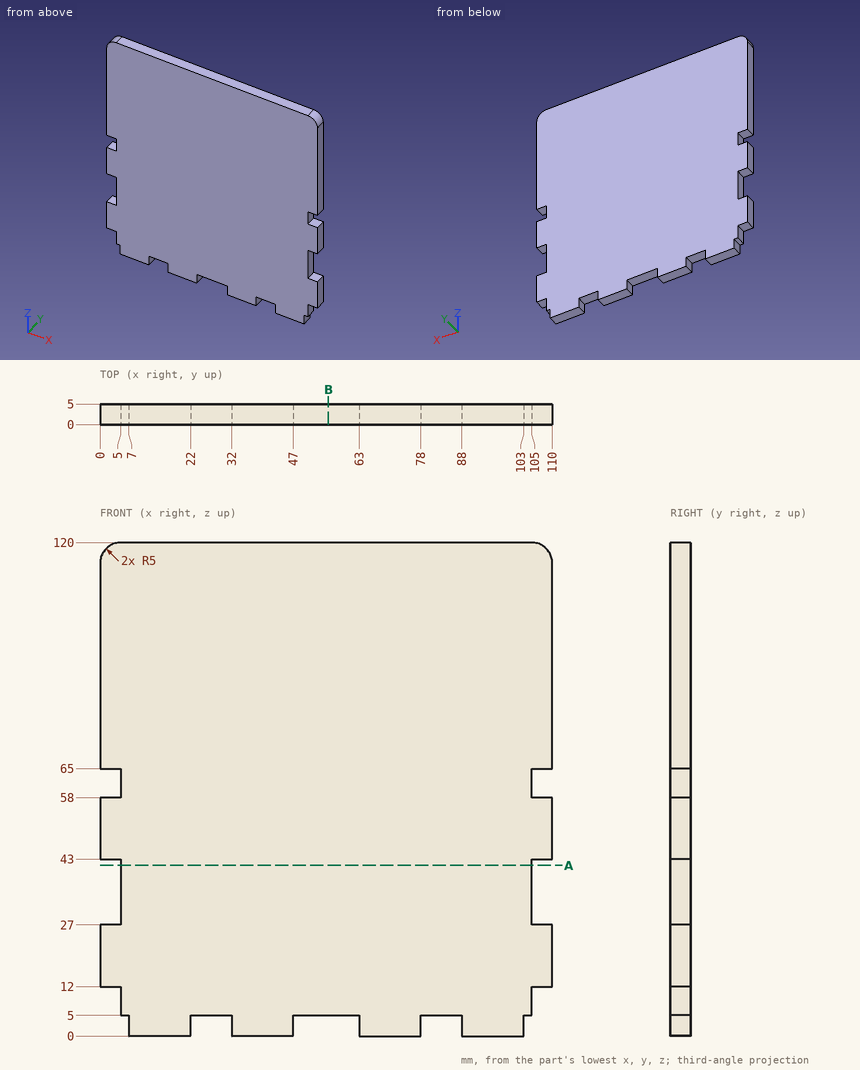
The figure shows three views and two pictorial views of one solid part (mm, origin at its lowest corner). Answer the questions. Give positions to 0.01 mm unless a question says otherwise; leave off trailing zeros. Loops run counter-clockwise (first coordinate to the right, second up) from the corner with the lowest first, then second, coordinate; pieces in that order, holes last. Notation, with made-up numbers: (41, 76) -> (68, 76) arc R18 cw to (68, 89) -> close; hole circle Ø2 at (51.25, -5.75). An arc over 180 degrees is marked (long way). Use a Markdown table: item, result. Add a question column.
1. Section A-A on z = 41.5 is taken. Determine the outline of the cut face in (x, y), and give its area (3 significant figures).
2. Flat-ended cylindrical pins translate along their axes: pin 1 Ø2.5 at (y, z) = (2.5, 3) entering from -X; pin 2 Ø1 at (x, y) = (104, 2.5) entering from -Z; pin 3 Ø1.5 at (y, z) = (2, 2) entering from +X. Find the tip coordinate at first contact, or state that the pin passes through.
3. Section B-B on x = 55.5 is taken. Determine the outline of the cut face in (y, z), and give its area (3 significant figures).
4. Find the intervals of material crossed by probe 1 along Z at (x, y) = (48.5, 4.3); probe 2 along X at (y, z) = (1.4, 10.5), in increasing order.
Results below:
| question | item | result |
|---|---|---|
| 1 | outline | (5, 0) -> (105, 0) -> (105, 5) -> (5, 5) -> close |
| 1 | area | 500 mm^2 |
| 2 | pin 1 | stops at x = 7 |
| 2 | pin 2 | stops at z = 5 |
| 2 | pin 3 | stops at x = 103 |
| 3 | outline | (0, 5) -> (5, 5) -> (5, 120) -> (0, 120) -> close |
| 3 | area | 575 mm^2 |
| 4 | probe 1 | z = 5 to 120 |
| 4 | probe 2 | x = 5 to 105 |
